Here's how the part is built. I have some questions about the finished solid (model axes, mm). Face numbers are marked on the shaded views. A direction names the side the tool comes from. Round coordinates to 2 decimals unless told otherwise and drop trailing zeros. Order: outer loops, then holes, each group sorted by start corner. A loop starts at its lowest first (then second) coordinate and runs counter-clockwise, first axis right, second up. Notation, with made-up numbers: (17.25, 79) -> (46.25, 79) arc R22 ccw to (46.25, 96) -> close; hole circle Ø6 at (86, -23.5). An arc over 180 degrees is marked (long way). Answer in a Markdown table with one row per item.
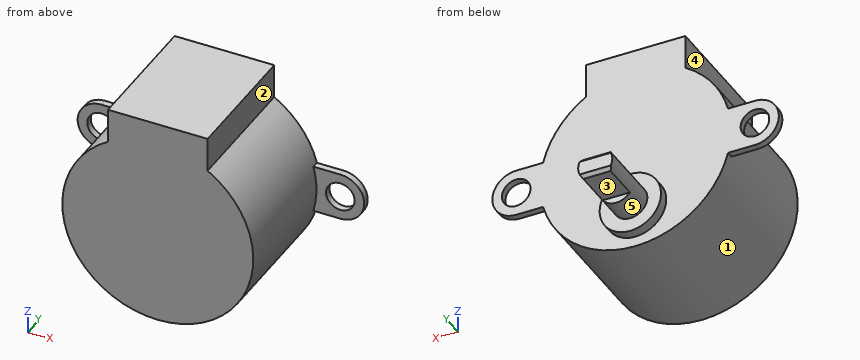
```python
from build123d import *

# Parameters (mm, degrees)
SKETCH1_R           = 14
BOSS_EXTRUDE1_DEPTH = 19
SKETCH2_R           = 2.1
BOSS_EXTRUDE2_DEPTH = 1
SKETCH3_R           = 4.5
BOSS_EXTRUDE3_DEPTH = 1.5
SKETCH4_R           = 2.5
BOSS_EXTRUDE4_DEPTH = 10
CUT_EXTRUDE1_DEPTH  = 6
CHAMFER1_SIZE       = 0.5
BOSS_EXTRUDE5_DEPTH = 19


with BuildPart() as part:
    # Sketch1 → Boss-Extrude1 (new body)
    with BuildSketch(Plane(origin=(0, 0, 0), x_dir=(1, 0, 0), z_dir=(0, 1, 0))):
        Circle(SKETCH1_R)
    extrude(amount=BOSS_EXTRUDE1_DEPTH)

    # Sketch2 → Boss-Extrude2 (add)
    with BuildSketch(Plane(origin=(0, 19, 0), x_dir=(1, 0, 0), z_dir=(0, 1, 0))):
        with BuildLine():
            Line((-17.5, 3.5), (-13.555441712, 3.5))
            ThreePointArc((-13.555441712, 3.5), (-14, 0), (-13.555441712, -3.5))
            Line((-13.555441712, -3.5), (-17.5, -3.5))
            ThreePointArc((-17.5, -3.5), (-21, 0), (-17.5, 3.5))
        make_face()
        with Locations((-17.5, 0)):
            Circle(SKETCH2_R, mode=Mode.SUBTRACT)
        with BuildLine():
            Line((17.5, -3.5), (13.555441712, -3.5))
            ThreePointArc((13.555441712, -3.5), (14, 0), (13.555441712, 3.5))
            Line((13.555441712, 3.5), (17.5, 3.5))
            ThreePointArc((17.5, 3.5), (21, 0), (17.5, -3.5))
        make_face()
        with Locations((17.5, 0)):
            Circle(SKETCH2_R, mode=Mode.SUBTRACT)
    extrude(amount=-BOSS_EXTRUDE2_DEPTH)

    # Sketch3 → Boss-Extrude3 (add)
    with BuildSketch(Plane(origin=(0, 19, 0), x_dir=(1, 0, 0), z_dir=(0, 1, 0))):
        with Locations((0, 8)):
            Circle(SKETCH3_R)
    extrude(amount=BOSS_EXTRUDE3_DEPTH)

    # Sketch4 → Boss-Extrude4 (add)
    with BuildSketch(Plane(origin=(0, 20.5, 0), x_dir=(1, 0, 0), z_dir=(0, 1, 0))):
        with Locations((0, 8)):
            Circle(SKETCH4_R)
    extrude(amount=BOSS_EXTRUDE4_DEPTH)

    # Sketch5 → Cut-Extrude1 (cut)
    with BuildSketch(Plane(origin=(0, 30.5, 0), x_dir=(1, 0, 0), z_dir=(0, 1, 0))):
        with BuildLine():
            Line((-2, 9.5), (2, 9.5))
            ThreePointArc((2, 9.5), (0, 10.5), (-2, 9.5))
        make_face()
        with BuildLine():
            Line((-2, 6.5), (2, 6.5))
            ThreePointArc((2, 6.5), (0, 5.5), (-2, 6.5))
        make_face()
    extrude(amount=-CUT_EXTRUDE1_DEPTH, mode=Mode.SUBTRACT)

    # Chamfer1
    chamfer1_edges = [part.edges().sort_by_distance(p)[0] for p in [
        (0, 30.5, -9.5),
        (0, 30.5, -6.5),
    ]]
    chamfer(chamfer1_edges, length=CHAMFER1_SIZE)

    # Sketch6 → Boss-Extrude5 (add)
    with BuildSketch(Plane(origin=(0, 19, 0), x_dir=(1, 0, 0), z_dir=(0, 1, 0))):
        with BuildLine():
            Line((-7.3, -17), (7.3, -17))
            Line((7.3, -17), (7.3, -11.94612908))
            ThreePointArc((7.3, -11.94612908), (0, -14), (-7.3, -11.94612908))
            Line((-7.3, -11.94612908), (-7.3, -17))
        make_face()
    extrude(amount=-BOSS_EXTRUDE5_DEPTH)


solid = part.part
```
1. Suppose I cut it at C-C on y = 23. Write out the boundary of the cut face in (x, z).
Numbers:
| item | result |
|---|---|
| outline | circle Ø5 at (0, -8) |
2. Suppose I cut it at B-B on z = 0. Write out the boundary of the cut face in (x, y), then the cut area to 3 significant figures.
Numbers:
| item | result |
|---|---|
| outline | (-21, 18) -> (-19.6, 18) -> (-19.6, 19) -> (-21, 19) -> close; (-15.4, 18) -> (-14, 18) -> (-14, 0) -> (14, 0) -> (14, 18) -> (15.4, 18) -> (15.4, 19) -> (-15.4, 19) -> close; (19.6, 18) -> (21, 18) -> (21, 19) -> (19.6, 19) -> close |
| area | 538 mm2 |
3. Suppose I cut it at D-D on z = -8. Write out the boundary of the cut face in (x, y), then the cut area to 3 significant figures.
Numbers:
| item | result |
|---|---|
| outline | (-11.49, 0) -> (11.49, 0) -> (11.49, 19) -> (4.5, 19) -> (4.5, 20.5) -> (2.5, 20.5) -> (2.5, 30.5) -> (-2.5, 30.5) -> (-2.5, 20.5) -> (-4.5, 20.5) -> (-4.5, 19) -> (-11.49, 19) -> close |
| area | 500 mm2 |
4. Suppose I cut it at A-A on x = 0. Write out the boundary of the cut face in (y, z), then the cut area to 3 significant figures.
Numbers:
| item | result |
|---|---|
| outline | (0, -14) -> (19, -14) -> (19, -12.5) -> (20.5, -12.5) -> (20.5, -10.5) -> (24.5, -10.5) -> (24.5, -9.5) -> (30, -9.5) -> (30.5, -9) -> (30.5, -7) -> (30, -6.5) -> (24.5, -6.5) -> (24.5, -5.5) -> (20.5, -5.5) -> (20.5, -3.5) -> (19, -3.5) -> (19, 17) -> (0, 17) -> close |
| area | 640 mm2 |
5. Please list where these lines run through material, in increasing order: line 1 along X through (y, z) = (18.45, 0); line 2 along Z through (x, y) = (17.5, 18.2); line 3 along Y through (x, z) = (-10.5, -8.5).
Numbers:
| item | result |
|---|---|
| line 1 | x = -21 to -19.6, -15.4 to 15.4, 19.6 to 21 |
| line 2 | z = -3.5 to -2.1, 2.1 to 3.5 |
| line 3 | y = 0 to 19 |
6. For pin 1 Ø1 at (x, y) = (-11.5, 14.5) entering from +Z; pin 2 Ø5 at (x, z) = (17.5, 0) entering from -Y; pin 3 Ø0.5 at (x, y) = (-15.5, 18.5) entering from +Z, each with a flat end and sliding along its axis, tell me the tip position at first contact or that it passes through.
Numbers:
| item | result |
|---|---|
| pin 1 | stops at z = 8.66 |
| pin 2 | stops at y = 18 |
| pin 3 | stops at z = 3.5 |
7. For the marked faces 1, 2, 3, 4 and 5, which set-ups out of +Z, -Z, +X, -X, +Y, -Y let a thin tool reach every point of the face, with its end or its side?
Numbers:
| item | result |
|---|---|
| face 1 | -Y |
| face 2 | +Z, +X, +Y, -Y |
| face 3 | -Z, +X, -X, +Y |
| face 4 | +Z, -X, +Y, -Y |
| face 5 | +Y |
